Geometry check sheet. Reference: the model listing, model coordinates, mm. A direction names the side the tool comes from. Give positions to 0.01 mm unless a question says otherwise; leave off trailing zeros. Answer as CSV lines item,"result".
from build123d import *

# Parameters (mm, degrees)
SKETCH_1_R          = 22
EXTRUDE_1_DEPTH     = 18.5
SKETCH_2_R          = 22
SKETCH_2_R_2        = 11
CUT_EXTRUDE_1_DEPTH = 4
SKETCH_4_R          = 22
SKETCH_4_RX         = 19.75
SKETCH_4_RY         = 19.5
CUT_EXTRUDE_2_DEPTH = 13
SKETCH_5_R          = 21.651989758
SKETCH_5_R_2        = 11
CUT_EXTRUDE_3_DEPTH = 4
CUT_EXTRUDE_4_DEPTH = 19.5
HOLE_WIZARD_1_1_D   = 3.9878
SKETCH_33_R         = 1.3
CUT_EXTRUDE_5_DEPTH = 2.5
CHAMFER_1_SIZE      = 0.3
CHAMFER_2_SIZE      = 0.2


with BuildPart() as part:
    # 草图1 → 凸台-拉伸1 (new body)
    with BuildSketch(Plane(origin=(0, 0, 0), x_dir=(1, 0, 0), z_dir=(0, 1, 0))):
        Circle(SKETCH_1_R)
    extrude(amount=EXTRUDE_1_DEPTH)

    # 草图2 → 切除-拉伸1 (cut)
    with BuildSketch(Plane(origin=(0, 18.5, 0), x_dir=(1, 0, 0), z_dir=(0, 1, 0))):
        Circle(SKETCH_2_R)
        Circle(SKETCH_2_R_2, mode=Mode.SUBTRACT)
    extrude(amount=-CUT_EXTRUDE_1_DEPTH, mode=Mode.SUBTRACT)

    # 草图4 → 切除-拉伸2 (cut)
    with BuildSketch(Plane.XZ):
        Circle(SKETCH_4_R)
        with Locations(Location((0, 0), (0, 0, 90))):
            Ellipse(SKETCH_4_RX, SKETCH_4_RY, mode=Mode.SUBTRACT)
    extrude(amount=-CUT_EXTRUDE_2_DEPTH, mode=Mode.SUBTRACT)

    # 草图5 → 切除-拉伸3 (cut)
    with BuildSketch(Plane.XZ):
        Circle(SKETCH_5_R)
        Circle(SKETCH_5_R_2, mode=Mode.SUBTRACT)
    extrude(amount=-CUT_EXTRUDE_3_DEPTH, mode=Mode.SUBTRACT)

    # 草图6 → 切除-拉伸4 (cut, through all)
    with BuildSketch(Plane(origin=(0, 18.5, 0), x_dir=(1, 0, 0), z_dir=(0, 1, 0))):
        with BuildLine():
            Line((-2.097599684, 8.471245207), (2.097599684, 8.471245207))
            Line((2.097599684, 8.471245207), (2.097599684, 6.415806697))
            ThreePointArc((2.097599684, 6.415806697), (0, -6.75), (-2.097599684, 6.415806697))
            Line((-2.097599684, 6.415806697), (-2.097599684, 8.471245207))
        make_face()
    extrude(amount=-CUT_EXTRUDE_4_DEPTH, mode=Mode.SUBTRACT)

    # #1 螺旋的螺纹孔钻头1 (through all)
    with Locations(Plane(origin=(0, 14.5, 0), x_dir=(1, 0, 0), z_dir=(0, 1, 0))):
        with Locations((0, 13.810288315), (-85.484743378, -69.881752856), (13.789919005, 0), (0, -13.801039256), (-13.69075507, 0)):
            Hole(HOLE_WIZARD_1_1_D / 2)

    # 草图33 → 切除-拉伸5 (cut)
    with BuildSketch(Plane(origin=(0, 18.5, 0), x_dir=(1, 0, 0), z_dir=(0, 1, 0))):
        with Locations((8.9, 0)):
            Circle(SKETCH_33_R)
        with Locations((-8.9, 0)):
            Circle(SKETCH_33_R)
    extrude(amount=-CUT_EXTRUDE_5_DEPTH, mode=Mode.SUBTRACT)

    # 倒角1
    chamfer_1_edges = [part.edges().sort_by_distance(p)[0] for p in [
        (-11.69685507, 4, 0),
        (-11.69685507, 14.5, 0),
        (1.9939, 4, 13.801039256),
        (1.9939, 14.5, 13.801039256),
        (15.783819005, 4, 0),
        (15.783819005, 14.5, 0),
        (1.9939, 4, -13.810288315),
        (1.9939, 14.5, -13.810288315),
    ]]
    chamfer(chamfer_1_edges, length=CHAMFER_1_SIZE)

    # 倒角2
    chamfer_2_edges = [part.edges().sort_by_distance(p)[0] for p in [
        (7.6, 18.5, 0),
        (-10.2, 18.5, 0),
    ]]
    chamfer(chamfer_2_edges, length=CHAMFER_2_SIZE)


solid = part.part
(1) Tool access check on faces 5 (the face through (-2.38, 1.97, -10.74)), 6 (the face through (-9, 16, 0)), 7 (the face through (0, 9, -8.471)). Record the directions out of +Z, -Z, +X, -X, +Y, -Y that give a thin tool (end or side, any length) a straight path to the whole face; none if there is none.
The answers:
face 5,"-Y"
face 6,"+Y"
face 7,"+Y, -Y"
(2) Gauge pin test, flat ends, axial feed: P1, Ø2, axis at x = 4, y = 14, coming from the -Z side; P2, Ø2, axis at x = 9.5, z = 0, coming from the +Y side; P3, Ø1.3, axis at x = 0, y = 13.5, coming from the +Z side; P4, Ø6, axis at x = 16.5, z = 7, coming from the -Y side. Record the tip position at first contact, or that the pin passes through.
The answers:
P1,"stops at z = -21.79"
P2,"stops at y = 18.5"
P3,"stops at z = 22"
P4,"stops at y = 4"
(3) Material ranges on line 1 (X direction, y = 9, z = 0); line 2 (X direction, y = 16.5, z = 0); line 3 (Y direction, x = -19, z = -6.5), recorded low to high.
The answers:
line 1,"x = -19.5 to -15.68, -11.7 to -6.75, 6.75 to 11.8, 15.78 to 19.5"
line 2,"x = -11 to -10.2, -7.6 to -6.75, 6.75 to 7.6, 10.2 to 11"
line 3,"y = 13 to 14.5"
(4) Draft check along X on faces 1 (the face through (-7.66, 17.17, -0.39)), 2 (the face through (-2.38, 16.53, 10.74)), 3 (the face through (-11.7, 9.2, -0.1)), 4 (the face through (-13, 13, 15)). Enter one of: +X half, -X half, draft (parallel to the pull), parting line (faces both ways), or undercut.
The answers:
face 1,"undercut"
face 2,"parting line"
face 3,"undercut"
face 4,"draft"
(5) Section check A-A on x = 0. State how many separate pieces and enclosed holes the cut face has, then the cut area to 3 significant figures.
The answers:
separate pieces,"4"
enclosed holes,"0"
area,"232 mm2"
